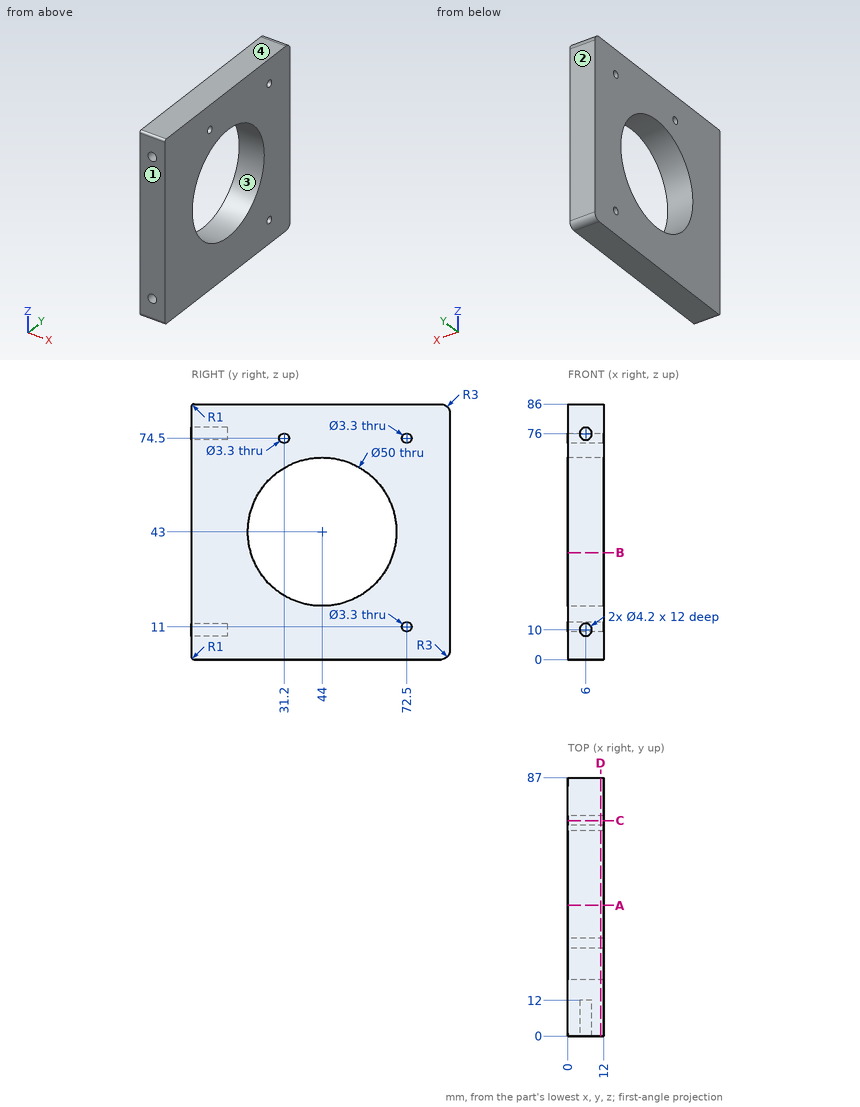
The drawing under review shows one solid part. Ordinate dimensions are in mm from its lowest x, y, z. Round coordinates to 2 decimals unless told otherwise and drop trailing zeros. Write each loop counter-clockwise with the first axis right and the second up, starting at its lowest first coordinate (ties: lowest second). Pieces come first, ordered by that corner, then holes. Notation, with made-up numbers: (39, 67.25) -> (93, 67.25) arc R10 cw to (93, 73.25) -> close; hole circle Ø8 at (79.25, 37.5). An arc over 180 degrees is marked (long way). Put each result on its own line as item: value.
Q1. Consider section B-B on z = 36. State the section outline as (x, y) points, and give its area (3 significant figures).
Determined:
outline: (0, 0) -> (12, 0) -> (12, 20) -> (0, 20) -> close; (0, 68) -> (12, 68) -> (12, 87) -> (0, 87) -> close
area: 468 mm^2
Q2. The part is to be moulded in two halves that separate along Y. For the marked faces 1, 2, 3 and 4, say which applies: released by +Y, released by -Y, zero draft, split by the parting line, or undercut.
Determined:
face 1: released by -Y
face 2: released by +Y
face 3: undercut
face 4: zero draft
Q3. Clearance check with a flat-ended pin moving along its axis: pin 1 Ø2 at (x, z) = (5.5, 9.5) entering from -Y. State where the tip first meets the part, or that it passes through.
Determined:
pin 1: stops at y = 12
Q4. Consider section A-A on y = 44. State the section outline as (x, z) points, and give its area (3 significant figures).
Determined:
outline: (0, 0) -> (12, 0) -> (12, 18) -> (0, 18) -> close; (0, 68) -> (12, 68) -> (12, 86) -> (0, 86) -> close
area: 432 mm^2
Q5. Consider section C-C on y = 72.5. State the section outline as (x, z) points.
Determined:
outline: (0, 0) -> (12, 0) -> (12, 9.35) -> (0, 9.35) -> close; (0, 12.65) -> (12, 12.65) -> (12, 72.85) -> (0, 72.85) -> close; (0, 76.15) -> (12, 76.15) -> (12, 86) -> (0, 86) -> close
Q6. To check wall thickness, follow L1, parallel to Z at x = 6, y = 3.5; L2, parallel to Y at x = 5.75, z = 74.5; L3, parallel to Z at x = 6.75, y = 72.5. State the ranges of each line that lie inside material, in increasing order. Write a range as [from, to].
Determined:
L1: z = [0, 7.9], [12.1, 73.9], [78.1, 86]
L2: y = [12, 29.55], [32.85, 70.85], [74.15, 87]
L3: z = [0, 9.35], [12.65, 72.85], [76.15, 86]
Q7. Consider section D-D on x = 11. State the section outline as (y, z) points, and give its area (3 significant figures).
Determined:
outline: (0, 1) arc R1 ccw to (1, 0) -> (84, 0) arc R3 ccw to (87, 3) -> (87, 83) arc R3 ccw to (84, 86) -> (1, 86) arc R1 ccw to (0, 85) -> close; hole circle Ø50 at (44, 43); hole circle Ø3.3 at (31.2, 74.5); hole circle Ø3.3 at (72.5, 11); hole circle Ø3.3 at (72.5, 74.5)
area: 5,490 mm^2
